Could you check a few things on this drawing? It's one solid part, dimensions in mm from its lowest x, y, z. Coordinates: 2 decimals unless noted, no trailing zeros. Order: outer loops, then holes, each group sorted by start corner. A loop starts at its lowest first (then second) coordinate and runs counter-clockwise, first axis right, second up. Notation, with made-up numbers: (-32.75, 35) - (26.25, 35) arc R18 cw to (26.25, 63) - close; hole circle Ø5 at (-36, 22). An arc over 180 degrees is marked (long way). Answer in a Markdown table with one row per item. Add a question column.
Item 1: I want a section at A-A (y = 1.4). Please give me the cut outline in (x, z) (3 decimals).
Item 2: If I drill on line 1 along Z through (x, y) = (59.5, 2); line 2 along Z through (x, y) = (93.5, 2.75), over which ranges is the centre line in solid material (lowest first)? Write a range as from..to.
Item 3: Will these pins go through, and if not, where does the flat tip stop? pin 1 Ø2 at (x, z) = (58, 97.5) entering from -Y; pin 2 Ø1 at (x, y) = (50.5, 2) entering from +Z.
Item 4: I want a section at B-B (x = 50). Please give me the cut outline in (y, z) (3 decimals), plus the area to 3 significant figures.
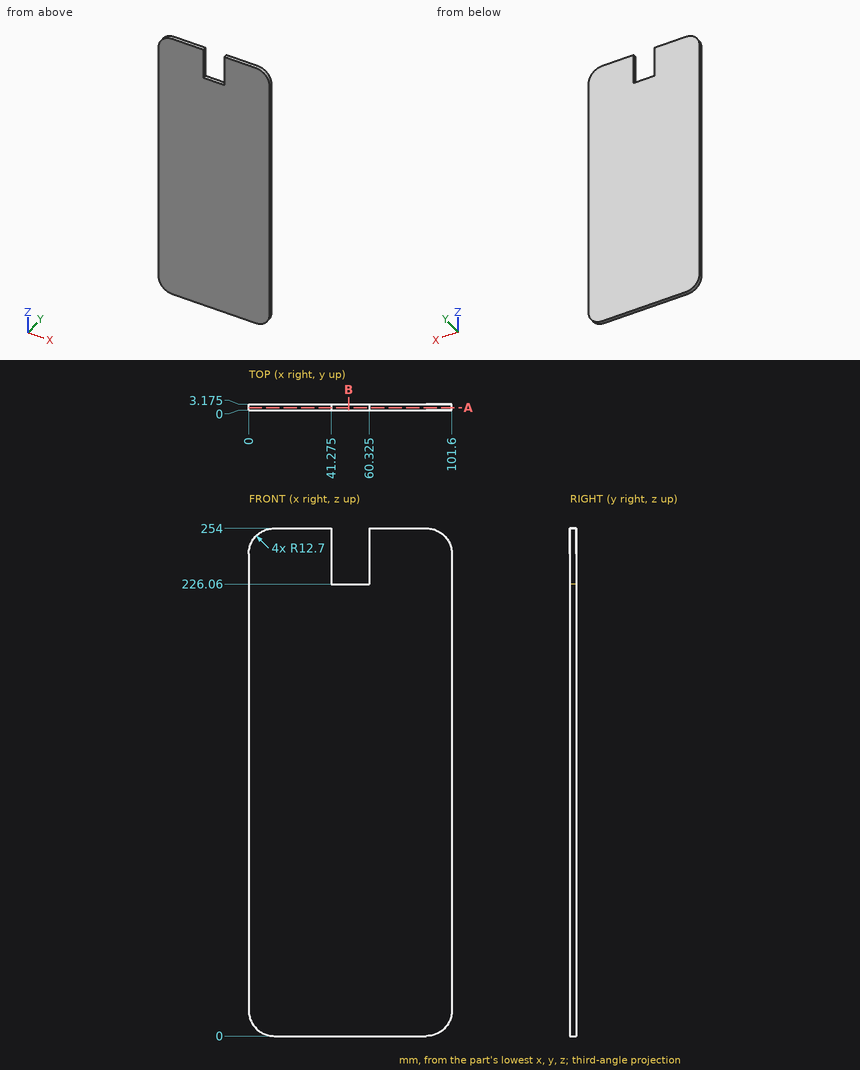
Values follow:
| question | item | result |
|---|---|---|
| 1 | outline | (0, 12.7) arc R12.7 ccw to (12.7, 0) - (88.9, 0) arc R12.7 ccw to (101.6, 12.7) - (101.6, 241.3) arc R12.7 ccw to (88.9, 254) - (60.325, 254) - (60.325, 226.06) - (41.275, 226.06) - (41.275, 254) - (12.7, 254) arc R12.7 ccw to (0, 241.3) - close |
| 2 | line 1 | z = 0..226.06 |
| 2 | line 2 | z = 0.86..253.14 |
| 3 | pin 1 | stops at y = 0 |
| 3 | pin 2 | stops at z = 226.06 |
| 4 | outline | (0, 0) - (3.175, 0) - (3.175, 226.06) - (0, 226.06) - close |
| 4 | area | 718 mm^2 |
